```python
from build123d import *

# Parameters (mm, degrees)
F1_DEPTH = 723.9
F2_SCALE = 0.125


with BuildPart() as f1:
    # F0 (on Right) → F1 (new body, symmetric)
    with BuildSketch(Plane.YZ):
        with BuildLine():
            Line((-15.8299067503, -142.596029821), (-11.8872214526, -143.0259399152))
            Line((-11.8872214526, -143.0259399152), (0, -18.7500006))
            Line((0, -18.7500006), (0, 18.7499994))
            Line((0, 18.7499994), (-7.9508239998, 58.7499994))
            ThreePointArc((-7.9508239998, 58.7499994), (-7.8920606963, 58.3597218998), (-7.8724079566, 57.9655348594))
            ThreePointArc((-7.8724079566, 57.9655348594), (-8.7715551646, 55.4519182766), (-11.0609952128, 54.0788930426))
            Line((-11.0609952128, 54.0788930426), (-3.9423238, 18.3539213456))
            Line((-3.9423238, 18.3539213456), (-11.835459815, 17.9655348594))
            Line((-11.835459815, 17.9655348594), (-11.835459815, 54.0024830011))
            ThreePointArc((-11.835459815, 54.0024830011), (-14.6385433533, 55.16401693), (-15.7985110549, 57.9677489647))
            Line((-15.7985110549, 57.9677489647), (-15.8207233853, 57.9655348594))
            Line((-15.8207233853, 57.9655348594), (-14.9394494697, -92.0344651406))
            Line((-14.9394494697, -92.0344651406), (-11.835459815, -12.0344651406))
            Line((-11.835459815, -12.0344651406), (-3.9423238, -12.0344651406))
            Line((-3.9423238, -12.0344651406), (-3.9423238, -18.5344211826))
            Line((-3.9423238, -18.5344211826), (-10.9737931654, -91.8188857231))
            Line((-10.9737931654, -91.8188857231), (-15.8299067503, -142.596029821))
        make_face()
        with BuildLine():
            ThreePointArc((-7.8724079566, 57.9655348594), (-7.8920606963, 58.3597218998), (-7.9508239998, 58.7499994))
            Line((-7.9508239998, 58.7499994), (-15.7985110549, 57.9677489647))
            ThreePointArc((-15.7985110549, 57.9677489647), (-14.6385433533, 55.16401693), (-11.835459815, 54.0024830011))
            Line((-11.835459815, 54.0024830011), (-11.835459815, 57.9655348594))
            Line((-11.835459815, 57.9655348594), (-11.0609952128, 54.0788930426))
            ThreePointArc((-11.0609952128, 54.0788930426), (-8.7715551646, 55.4519182766), (-7.8724079566, 57.9655348594))
        make_face()
        with BuildLine():
            Line((-15.7985110549, 57.9677489647), (-7.9508239998, 58.7499994))
            ThreePointArc((-7.9508239998, 58.7499994), (-12.2285452772, 61.9090439379), (-15.7985110549, 57.9677489647))
        make_face()
    extrude(amount=F1_DEPTH, both=True)


with BuildPart() as f1_1:
    # F2: moved
    add(f1.part.scale(F2_SCALE))


solid = f1_1.part
```
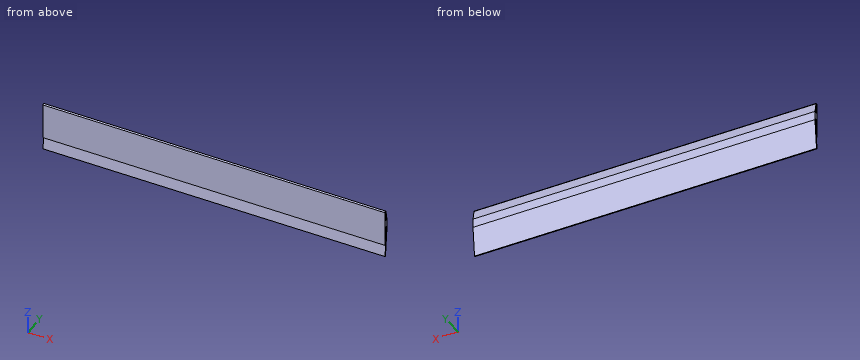
The listing builds one solid part. Answer for the finished solid, in the listing's coordinates (mm). Give positions to 0.01 mm unless a question says otherwise; leave off trailing zeros. Order: outer loops, then holes, each group sorted by start corner. A loop starts at its lowest first (then second) coordinate and runs counter-clockwise, first axis right, second up. Notation, with made-up numbers: M -38.5,34 L -7.5,34 A13 cw -7.5,55 Z; hole C 86.25,78.25 d2. An arc over 180 degrees is marked long. Put each result on its own line as item: value. Start each with the question number.
Item 1: Flat-ended cylindrical pins translate along their axes: P1, Ø1, axis at x = -37.5, z = -13.5, coming from the -Y side; P2, Ø1.5, axis at x = 29, z = 4, coming from the +Y side; P3, Ø1, axis at x = 36, z = -15, coming from the -Y side. Find the tip coordinate at first contact, or state that the pin passes through.
Item 2: The part is cut by section C-C, the plane z = -15.75. Determine the outline of the cut face in (x, y), and give its area (3 significant figures).
Item 3: Find the intervals of material crossed by line 1 along Y through (x, z) = (-39, 4.75); line 2 along Y through (x, z) = (57.5, -6.5); line 3 along Y through (x, z) = (-0.5, 2), in increasing order.
Item 4: The part is cut by section B-B, the plane z = 4.75. Determine the outline of the cut face in (x, y), and give its area (3 significant figures).
Answer key:
1. P1: stops at y = -1.61
1. P2: stops at y = -0.18
1. P3: stops at y = -1.76
2. outline: M -90.49,-1.78 L 90.49,-1.78 L 90.49,-1.28 L -90.49,-1.28 Z
2. area: 90.1 mm²
3. line 1: y = -1.96 to -1.48, -0.98 to -0.48
3. line 2: y = -1.9 to -1.67, -0.89 to -0.4
3. line 3: y = -1.95 to 0
4. outline: M -90.49,-1.96 L 90.49,-1.96 L 90.49,-1.48 L -90.49,-1.48 Z; M -90.49,-0.98 L 90.49,-0.98 L 90.49,-0.48 L -90.49,-0.48 Z
4. area: 179 mm²
